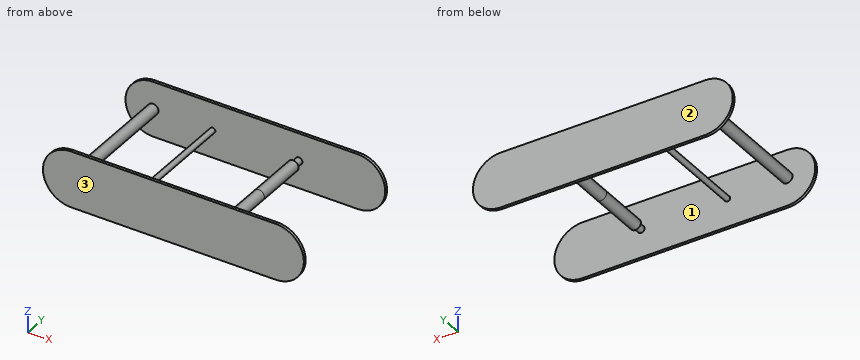
from build123d import *

# Parameters (mm, degrees)
BOSS_EXTRUDE1_DEPTH = 3.2
SKETCH8_R           = 6.15
BOSS_EXTRUDE5_DEPTH = 140
BOSS_EXTRUDE6_DEPTH = 3.2
SKETCH12_R          = 3
BOSS_EXTRUDE7_DEPTH = 140
SKETCH14_R          = 3.9
BOSS_EXTRUDE8_DEPTH = 10
SKETCH15_R          = 6.15
BOSS_EXTRUDE9_DEPTH = 60


with BuildPart() as part:
    # Sketch1 → Boss-Extrude1 (new body)
    with BuildSketch(Plane(origin=(0, 0, 0), x_dir=(1, 0, 0), z_dir=(0, 1, 0))):
        with BuildLine():
            Line((-110.589063221, 31.6), (119.210936779, 31.6))
            ThreePointArc((119.210936779, 31.6), (150.810936779, 0), (119.210936779, -31.6))
            Line((119.210936779, -31.6), (-110.589063221, -31.6))
            ThreePointArc((-110.589063221, -31.6), (-142.189063221, 0), (-110.589063221, 31.6))
        make_face()
    extrude(amount=BOSS_EXTRUDE1_DEPTH)

    # Sketch8 → Boss-Extrude5 (add)
    with BuildSketch(Plane(origin=(0, 3.2, 0), x_dir=(1, 0, 0), z_dir=(0, 1, 0))):
        with Locations(Location((-110.589063221, 0, 0), (0, 0, 270))):
            Circle(SKETCH8_R)
    extrude(amount=BOSS_EXTRUDE5_DEPTH)

    # Sketch11 → Boss-Extrude6 (add)
    with BuildSketch(Plane(origin=(0, 143.2, 0), x_dir=(1, 0, 0), z_dir=(0, 1, 0))):
        with BuildLine():
            Line((-110.589063221, 30.988193708), (119.210936779, 30.988193708))
            ThreePointArc((119.210936779, 30.988193708), (150.199130487, 0), (119.210936779, -30.988193708))
            Line((119.210936779, -30.988193708), (-110.589063221, -30.988193708))
            ThreePointArc((-110.589063221, -30.988193708), (-141.577256929, 0), (-110.589063221, 30.988193708))
        make_face()
    extrude(amount=BOSS_EXTRUDE6_DEPTH)

    # Sketch12 → Boss-Extrude7 (add)
    with BuildSketch(Plane(origin=(0, 3.2, 0), x_dir=(1, 0, 0), z_dir=(0, 1, 0))):
        with Locations(Location((-43.639063221, 0, 0), (0, 0, 270))):
            Circle(SKETCH12_R)
    extrude(amount=BOSS_EXTRUDE7_DEPTH)

    # Sketch14 → Boss-Extrude8 (add)
    with BuildSketch(Plane(origin=(0, 3.2, 0), x_dir=(1, 0, 0), z_dir=(0, 1, 0))):
        with Locations(Location((53.310936779, 0, 0), (0, 0, 270))):
            Circle(SKETCH14_R)
    boss_extrude8 = extrude(amount=BOSS_EXTRUDE8_DEPTH)

    # Sketch15 → Boss-Extrude9 (add)
    with BuildSketch(Plane(origin=(0, 13.2, 0), x_dir=(1, 0, 0), z_dir=(0, 1, 0))):
        with Locations(Location((53.310936779, 0, 0), (0, 0, 270))):
            Circle(SKETCH15_R)
    boss_extrude9 = extrude(amount=BOSS_EXTRUDE9_DEPTH)

    # Mirror7: Boss-Extrude8, Boss-Extrude9 across plane
    add(boss_extrude8.mirror(Plane.ZX.offset(73.2)))
    add(boss_extrude9.mirror(Plane.ZX.offset(73.2)))


solid = part.part
Design review of the part built by this model. Coordinates are the model's own, in mm. Face numbers are marked on the shaded views. Coordinates: 2 decimals unless noted, no trailing zeros. Loops run counter-clockwise (first coordinate to the right, second up) from the corner with the lowest first, then second, coordinate; pieces in that order, holes last. Notation, with made-up numbers: M 20,80.25 L 26,80.25 A22 ccw 26,102.25 Z; hole C -21,46.25 d11. An arc over 180 degrees is marked long. Answer as CSV lines item,"result".
Item 1: Add section C-C on z = 0. State the section outline as (x, y) points.
Answer list:
outline,"M -142.19,0 L 150.81,0 L 150.81,3.2 L 57.21,3.2 L 57.21,13.2 L 59.46,13.2 L 59.46,133.2 L 57.21,133.2 L 57.21,143.2 L 150.2,143.2 L 150.2,146.4 L -141.58,146.4 L -141.58,143.2 L -116.74,143.2 L -116.74,3.2 L -142.19,3.2 Z; hole M -104.44,3.2 L -46.64,3.2 L -46.64,143.2 L -104.44,143.2 Z; hole M -40.64,3.2 L 49.41,3.2 L 49.41,13.2 L 47.16,13.2 L 47.16,133.2 L 49.41,133.2 L 49.41,143.2 L -40.64,143.2 Z"
Item 2: The part is to be moulded in two halves that separate along Y. For the marked faces 1, 2 and 3, say which applies: pulls with the +Y half, pulls with the -Y half, needs draft (parallel to the pull), parting line crosses it, or undercut.
Answer list:
face 1,"undercut"
face 2,"pulls with the +Y half"
face 3,"pulls with the -Y half"
Item 3: For probe 1 along Y at (x, z) = (58, 2.5); probe 2 along Y at (x, z) = (48, 21.5); probe 3 along X at (y, z) = (37, 1), list the stretches that pass through material, from the lowest coordinate up.
Answer list:
probe 1,"0 to 3.2, 13.2 to 133.2, 143.2 to 146.4"
probe 2,"0 to 3.2, 143.2 to 146.4"
probe 3,"-116.66 to -104.52, -46.47 to -40.81, 47.24 to 59.38"
Item 4: Add section D-D on y = 43. State the section outline as (x, z) points, plus the area to 3 significant figures.
Answer list:
outline,"C -110.59,0 d12.3; C -43.64,0 d6; C 53.31,0 d12.3"
area,"266 mm²"
Item 5: Add section A-A on x = 24. State the section outline as (y, z) points, plus the area to 3 significant figures.
Answer list:
outline,"M 0,-31.6 L 3.2,-31.6 L 3.2,31.6 L 0,31.6 Z; M 143.2,-30.99 L 146.4,-30.99 L 146.4,30.99 L 143.2,30.99 Z"
area,"401 mm²"
Item 6: For P1, Ø1, axis at x = -21.5, y = 145, coming from the +Z side; P2, Ø3.5, axis at x = -43, y = 144, coming from the -Z side, all flat-tipped, find the tip position at first contact; note any pin that passes through.
Answer list:
P1,"z = 30.99"
P2,"z = -30.99"
Item 7: Add section B-B on z = 25. State the section outline as (x, y) points, plus the area to 3 significant figures.
Answer list:
outline,"M -129.92,0 L 138.54,0 L 138.54,3.2 L -129.92,3.2 Z; M -128.9,143.2 L 137.52,143.2 L 137.52,146.4 L -128.9,146.4 Z"
area,"1,710 mm²"
